Autodesk Inventor part; units mm, degrees
ref_plane "YZ Plane" through (0, 0, 0) normal (1, 0, 0) x (0, 1, 0)
ref_plane "XZ Plane" through (0, 0, 0) normal (0, 1, 0) x (-1, 0, 0)
ref_plane "XY Plane" through (0, 0, 0) normal (0, 0, 1) x (1, 0, 0)
sketch "Sketch1" plane through (0, 0, 0) normal (0, 0, 1) x (1, 0, 0)
  line L0 (0, 0) -> (0, 40.5892) construction
  line L1 (0, 0) -> (0, -19.05) construction
  circle A0 centre (0, 40.5892) radius 11
  line L2 (-15.5, 25.0892) -> (15.5, 25.0892) construction
  line L3 (15.5, 25.0892) -> (15.5, 56.0892) construction
  line L4 (15.5, 56.0892) -> (-15.5, 56.0892) construction
  line L5 (-15.5, 56.0892) -> (-15.5, 25.0892) construction
  line L6 (-15.5, 25.0892) -> (15.5, 56.0892) construction
  line L7 (15.5, 25.0892) -> (-15.5, 56.0892) construction
  line L8 (-21, 20.0892) -> (21, 20.0892) construction
  line L9 (21, 21.2575) -> (21, 57.9142)
  line L10 (17.825, 61.0892) -> (-17.825, 61.0892)
  line L11 (-21, 57.9142) -> (-21, 21.2575)
  line L12 (-21, 20.0892) -> (21, 61.0892) construction
  line L13 (21, 20.0892) -> (-21, 61.0892) construction
  line L14 (0, -19.05) -> (0, -38.1) construction
  line L15 (19.05, -19.05) -> (38.1, -19.05) construction
  line L16 (-19.05, -19.05) -> (-38.1, -19.05) construction
  line L17 (-34.925, -38.1) -> (34.925, -38.1)
  line L18 (38.1, -34.925) -> (38.1, -1.1683)
  line L19 (38.1, 0) -> (-38.1, 0) construction
  line L20 (-38.1, -1.1683) -> (-38.1, -34.925)
  line L21 (-21.7573, 19.1995) -> (-37.3427, 0.8897)
  line L22 (21.7573, 19.1995) -> (37.3427, 0.8897)
  arc A1 (-17.825, 61.0892) -> (-21, 57.9142) centre (-17.825, 57.9142) ccw
  arc A2 (-21.7573, 19.1995) -> (-21, 21.2575) centre (-24.175, 21.2575) ccw
  arc A3 (21, 21.2575) -> (21.7573, 19.1995) centre (24.175, 21.2575) ccw
  arc A4 (38.1, -1.1683) -> (37.3427, 0.8897) centre (34.925, -1.1683) ccw
  arc A5 (34.925, -38.1) -> (38.1, -34.925) centre (34.925, -34.925) ccw
  arc A6 (-38.1, -34.925) -> (-34.925, -38.1) centre (-34.925, -34.925) ccw
  arc A7 (-37.3427, 0.8897) -> (-38.1, -1.1683) centre (-34.925, -1.1683) ccw
  arc A8 (21, 57.9142) -> (17.825, 61.0892) centre (17.825, 57.9142) ccw
  point P0 (-38.1, -38.1)
  point P1 (38.1, -38.1)
  dimension "d0" = 40.5892
  dimension "d1" = 19.05
  dimension "d2" = 22
  dimension "d3" = 31
  dimension "d4" = 31
  dimension "d5" = 42
  dimension "d6" = 41
  dimension "d10" = 19.05
  dimension "d11" = 19.05
  dimension "d12" = 19.05
  dimension "d13" = 19.05
  dimension "d14" = 19.05
  dimension "d15" = 19.05
  dimension "d16" = 19.05
  dimension "d17" = 76.2
  dimension "d18" = 19.05
  dimension "d19" = 19.05
  dimension "d20" = 38.1
  dimension "d22" = 38.1
  dimension "d23" = 3.175
  dimension "d24" = 3.175
  dimension "d25" = 3.175
extrude "Extrusion1" add sketch "Sketch1" along normal blind 3.175
hole "Hole1" at (0, -19.05, 0) at (0, 40.5892, 0) at (19.05, -19.05, 0) at (-19.05, -19.05, 0) direction (0, 0, 1) diameter 6.7564 end through all
hole "Hole2" at (-15.5, 56.0892, 0) at (-15.5, 25.0892, 0) at (15.5, 25.0892, 0) at (15.5, 56.0892, 0) direction (0, 0, 1) diameter 3.4036 end through all
properties part number "y_motor_mount"
Can you work these out from the model? Positions are in its coordinate system, mm. A direction names the side the tool comes from. Give positions to 0.01 mm unless a question says otherwise; leave off trailing zeros. Write each loop counter-clockwise with the first axis right and the second up, starting at its lowest first coordinate (ties: lowest second). Pieces come first, ordered by that corner, then holes. Notation, with made-up numbers: (24, 27) -> (38, 27) arc R17 ccw to (38, 44) -> close; hole circle Ø5 at (39.5, -12). An arc over 180 degrees is marked (long way). Answer as a JSON object with one key per item and string values. Group by question number.
Item 1: I'm going to push flat-ended pins straight in: P1, Ø8, axis at x = 0, y = -19.05, coming from the -Z side; P2, Ø20, axis at x = 0, y = 40.59, coming from the -Z side; P3, Ø1, axis at y = 40.5, z = 2, coming from the -X side; P4, Ø1.6, axis at y = 46.5, z = 2.5, coming from the +X side. Where does each tip first touch, or does it pass through?
Item 2: Suppose I cut it at D-D (y = 13). Please give me the cut outline in (x, z) (3 decimals).
Item 3: Suppose I cut it at C-C (x = -19.05). Please give me the cut outline in (y, z) (3 decimals), plus the area to 3 significant figures.
Item 4: For faces 1 (the face through (-29.441, 10.173, 1.565)), 2 (the face through (21, 39, 2)), which set-ups out of +Z, -Z, +X, -X, +Y, -Y let a thin tool reach every point of the face, with its end or its side?
Item 5: We'd pull the mould along Y, two halves only. Please class faces 3 (the face through (15.7, -19.5, 1.6)), 4 (the face through (-21, 40, 2)), 5 (the face through (-37.91, -0.09, 1.57)): +Y half, -Y half, draft (parallel to the pull), parting line (faces both ways), or undercut.
Item 6: Suppose I cut it at A-A (y = -19.05). Please give me the cut outline in (x, z) (3 decimals).
Item 7: Suppose I cut it at B-B (z = 1.9). State how many separate pieces and enclosed holes the cut face has, plus the area to 3 significant figures.
Item 8: Please list where these lines run through material, in increasing order: line 1 (Y direction, x = -15.5, z = 0.8); line 2 (Y direction, x = 0, z = 0.9); line 3 (X direction, y = -18.5, z = 2). Write a range as [from, to].
Findings:
{
 "1": {"P1": "stops at z = 0", "P2": "passes through", "P3": "stops at x = -21", "P4": "stops at x = 21"},
 "2": {"outline": "(-27.034, 0) -> (27.034, 0) -> (27.034, 3.175) -> (-27.034, 3.175) -> close"},
 "3": {"outline": "(-38.1, 0) -> (-22.428, 0) -> (-22.428, 3.175) -> (-38.1, 3.175) -> close; (-15.672, 0) -> (60.843, 0) -> (60.843, 3.175) -> (-15.672, 3.175) -> close", "area": "293 mm²"},
 "4": {"face 1": "+Z, -Z, -X, +Y", "face 2": "+Z, -Z, +X, +Y"},
 "5": {"face 3": "undercut", "face 4": "draft", "face 5": "+Y half"},
 "6": {"outline": "(-38.1, 0) -> (-22.428, 0) -> (-22.428, 3.175) -> (-38.1, 3.175) -> close; (-15.672, 0) -> (-3.378, 0) -> (-3.378, 3.175) -> (-15.672, 3.175) -> close; (3.378, 0) -> (15.672, 0) -> (15.672, 3.175) -> (3.378, 3.175) -> close; (22.428, 0) -> (38.1, 0) -> (38.1, 3.175) -> (22.428, 3.175) -> close"},
 "7": {"separate pieces": "1", "enclosed holes": "8", "area": "5,280 mm²"},
 "8": {"line 1": "y = [-38.1, 23.39], [26.79, 54.39], [57.79, 61.09]", "line 2": "y = [-38.1, -22.43], [-15.67, 29.59], [51.59, 61.09]", "line 3": "x = [-38.1, -22.38], [-15.72, -3.33], [3.33, 15.72], [22.38, 38.1]"}
}
